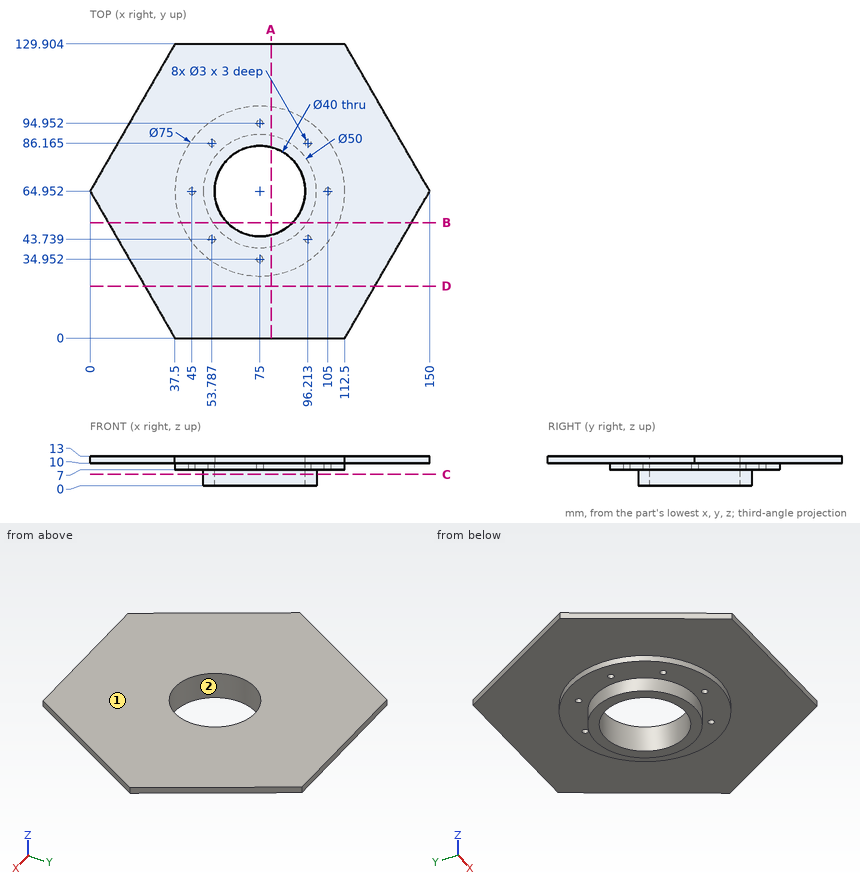
Study the drawing (mm; zero at the part's minimum x, y, z) and answer. Coordinates: 2 decimals unless noted, no trailing zeros. Loops run counter-clockwise (first coordinate to the right, second up) from the corner with the lowest first, then second, coordinate; pieces in that order, holes last. Notation, with made-up numbers: (22, 20) -> (75, 20) arc R24 ccw to (75, 59) -> close; hole circle Ø4 at (17, 6). An arc over 180 degrees is marked (long way). Answer in a Markdown table with one row per item. Add a question column.
1. Determine the mould class of the marked faces 1 and 2 for opening direction Y: +Y half, -Y half, draft (parallel to the pull), parting line (faces both ways), or undercut.
2. The part is cut by section C-C, the plane z = 5. Write down the section's boundary in (x, y), then the cut area to 3 significant figures.
3. The part is cut by section D-D, the plane y = 23. Write down the section's boundary in (x, z).
4. The part is cut by section B-B, the plane y = 51. Write down the section's boundary in (x, z) (1 decimal).
5. Consider line 1 (Y direction, x = 75, z = 8.35); line 2 (Z direction, x = 123, y = 98); line 3 (Y direction, x = 70, z = 2.5). Determine where each line is inside the solid, lowest interval first. Write a range as [from, to].
6. The part is cut by section A-A, the plane x = 80. Write down the section's boundary in (y, z), then the cut area to 3 significant figures.
7. Flat-ended cylindrical pins translate along their axes: P1, Ø3.5, axis at x = 44.5, y = 65, coming from the -Z side; P2, Ø2.5, axis at x = 45, y = 64.95, coming from the -Z side; P3, Ø24, axis at x = 75, y = 64.95, coming from the -Z side; P4, Ø6, axis at y = 78, z = 2.5, coming from the +X side. Find the tip coordinate at first contact, or state that the pin passes through.
Answer below:
| question | item | result |
|---|---|---|
| 1 | face 1 | draft |
| 1 | face 2 | undercut |
| 2 | outline | circle Ø50 at (75, 64.95); hole circle Ø40 at (75, 64.95) |
| 2 | area | 707 mm2 |
| 3 | outline | (24.22, 10) -> (125.78, 10) -> (125.78, 13) -> (24.22, 13) -> close |
| 4 | outline | (8.1, 10) -> (40.2, 10) -> (40.2, 7) -> (54.3, 7) -> (54.3, 0) -> (60.7, 0) -> (60.7, 13) -> (8.1, 13) -> close; (89.3, 0) -> (95.7, 0) -> (95.7, 7) -> (109.8, 7) -> (109.8, 10) -> (141.9, 10) -> (141.9, 13) -> (89.3, 13) -> close |
| 5 | line 1 | [27.45, 33.45], [36.45, 44.95], [84.95, 93.45], [96.45, 102.45] |
| 5 | line 2 | [10, 13] |
| 5 | line 3 | [40.46, 45.59], [84.32, 89.45] |
| 6 | outline | (0, 10) -> (27.79, 10) -> (27.79, 7) -> (40.46, 7) -> (40.46, 0) -> (45.59, 0) -> (45.59, 13) -> (0, 13) -> close; (84.32, 0) -> (89.45, 0) -> (89.45, 7) -> (102.12, 7) -> (102.12, 10) -> (129.9, 10) -> (129.9, 13) -> (84.32, 13) -> close |
| 6 | area | 452 mm2 |
| 7 | P1 | z = 7 |
| 7 | P2 | z = 10 |
| 7 | P3 | through |
| 7 | P4 | x = 97.89 |
